Could you check a few things on this model? Use its own coordinates, in mm. A direction names the side the tool comes from. Round coordinates to 2 decimals unless told otherwise and drop trailing zeros. Loops run counter-clockwise (first coordinate to the right, second up) from the corner with the lowest first, then second, coordinate; pieces in that order, holes last. Notation, with made-up numbers: (1, -11) - (58, -11) arc R22 cw to (58, -1) - close; hole circle Ø11 at (20.25, 1). An arc over 180 degrees is marked (long way). Use one line per item in the form item = value.
```python
from build123d import *

# Parameters (mm, degrees)
SKETCH1_W           = 1300
SKETCH1_H           = 300
BOSS_EXTRUDE1_DEPTH = 700
FILLET1_R           = 200
FILLET2_R           = 100
FILLET3_R           = 100
FILLET4_R           = 100
SKETCH3_R           = 3.4
CUT_EXTRUDE1_DEPTH  = 100
CUT_EXTRUDE2_START  = -100
SKETCH4_R           = 3.4
CUT_EXTRUDE2_DEPTH  = 100
SKETCH5_W           = 631.976111166
SKETCH5_H           = 319.581114146
CUT_EXTRUDE4_DEPTH  = 1410
SKETCH6_W           = 352.69600487
SKETCH6_H           = 35.021102412
BOSS_EXTRUDE2_DEPTH = 631.976111165


with BuildPart() as part:
    # Sketch1 → Boss-Extrude1 (new body)
    with BuildSketch(Plane(origin=(0, 0, 0), x_dir=(-1, 0, 0), z_dir=(0, 1, 0))):
        Rectangle(SKETCH1_W, SKETCH1_H)
    extrude(amount=BOSS_EXTRUDE1_DEPTH)

    # Fillet1
    fillet1_edges = [part.edges().sort_by_distance(p)[0] for p in [
        (650, 350, 150),
    ]]
    fillet(fillet1_edges, radius=FILLET1_R)

    # Fillet2
    fillet2_edges = [part.edges().sort_by_distance(p)[0] for p in [
        (650, 350, -150),
    ]]
    fillet(fillet2_edges, radius=FILLET2_R - 0.0001)  # a hair under: the kernel refuses the full size

    # Fillet3
    fillet3_edges = [part.edges().sort_by_distance(p)[0] for p in [
        (-650, 350, 150),
    ]]
    fillet(fillet3_edges, radius=FILLET3_R)

    # Fillet4
    fillet4_edges = [part.edges().sort_by_distance(p)[0] for p in [
        (-650, 350, -150),
    ]]
    fillet(fillet4_edges, radius=FILLET4_R)

    # Sketch3 → Cut-Extrude1 (cut)
    with BuildSketch(Plane.XZ):
        with Locations(Location((475, 0, 0), (0, 0, 270))):
            Circle(SKETCH3_R)
        with Locations(Location((492.320508076, 10, 0), (0, 0, 270))):
            Circle(SKETCH3_R)
        with Locations(Location((457.679491924, 10, 0), (0, 0, 270))):
            Circle(SKETCH3_R)
        with Locations(Location((475, -20, 0), (0, 0, 270))):
            Circle(SKETCH3_R)
        with Locations(Location((-475, 0, 0), (0, 0, 270))):
            Circle(SKETCH3_R)
        with Locations(Location((-457.679491924, 10, 0), (0, 0, 270))):
            Circle(SKETCH3_R)
        with Locations(Location((-492.320508076, 10, 0), (0, 0, 270))):
            Circle(SKETCH3_R)
        with Locations(Location((-475, -20, 0), (0, 0, 270))):
            Circle(SKETCH3_R)
    extrude(amount=-CUT_EXTRUDE1_DEPTH, mode=Mode.SUBTRACT)

    # Sketch4 → Cut-Extrude2 (cut)
    with BuildSketch(Plane(origin=(0, 700, 0), x_dir=(-1, 0, 0), z_dir=(0, 1, 0)).offset(CUT_EXTRUDE2_START)):
        with Locations(Location((-475, 0, 0), (0, 0, 270))):
            Circle(SKETCH4_R)
        with Locations(Location((-475, 20, 0), (0, 0, 90))):
            Circle(SKETCH4_R)
        with Locations(Location((-492.320508076, -10, 0), (0, 0, 90))):
            Circle(SKETCH4_R)
        with Locations(Location((-457.679491924, -10, 0), (0, 0, 90))):
            Circle(SKETCH4_R)
        with Locations(Location((475, 0, 0), (0, 0, 270))):
            Circle(SKETCH4_R)
        with Locations(Location((475, 20, 0), (0, 0, 90))):
            Circle(SKETCH4_R)
        with Locations(Location((457.679491924, -10, 0), (0, 0, 90))):
            Circle(SKETCH4_R)
        with Locations(Location((492.320508076, -10, 0), (0, 0, 90))):
            Circle(SKETCH4_R)
    extrude(amount=CUT_EXTRUDE2_DEPTH, mode=Mode.SUBTRACT)

    # Sketch5 → Cut-Extrude4 (cut)
    with BuildSketch(Plane(origin=(-650, 0, 0), x_dir=(0, -1, 0), z_dir=(-1, 0, 0))):
        with Locations((-350, -43.959211894)):
            Rectangle(SKETCH5_W, SKETCH5_H)
    extrude(amount=-CUT_EXTRUDE4_DEPTH, mode=Mode.SUBTRACT)

    # Sketch6 → Boss-Extrude2 (add)
    with BuildSketch(Plane(origin=(0, 34.011944417, 0), x_dir=(-1, 0, 0), z_dir=(0, 1, 0))):
        with Locations((26.80489637, -132.489448794)):
            Rectangle(SKETCH6_W, SKETCH6_H)
    extrude(amount=BOSS_EXTRUDE2_DEPTH)


solid = part.part
```
1. We'd pull the mould along Y, two halves only. Please class faces 1 (the face through (8, 267, -150)), 2 (the face through (9, 0, 2)), 3 (the face through (-9, 665.988, -19)), 4 (the face through (9, 700, 2)): +Y half, -Y half, draft (parallel to the pull), parting line (faces both ways), or undercut.
Solution:
face_1 = draft
face_2 = -Y half
face_3 = undercut
face_4 = +Y half
2. For P1, Ø6, axis at x = -457.68, z = 10, coming from the -Y side; P2, Ø4, axis at x = 475, z = 0, coming from the -Y side; P3, Ø10.5, axis at y = 341.5, z = -125, coming from the -X side, each with a flat end and sliding along its axis, tell me the tip position at first contact or that it passes through.
Solution:
P1 = 665.99
P2 = through
P3 = -203.15
3. If we section it at D-D, the plane x = -168: Write out the boundary of the cut face in (y, z).
Solution:
outline = (0, -150) - (700, -150) - (700, 150) - (0, 150) - close; hole (34.01, -114.98) - (665.99, -114.98) - (665.99, 115.83) - (34.01, 115.83) - close
4. If we section it at C-C, the plane x = 301.5: Write out the boundary of the cut face in (y, z).
Solution:
outline = (0, -150) - (34.01, -150) - (34.01, 115.83) - (665.99, 115.83) - (665.99, -150) - (700, -150) - (700, 150) - (0, 150) - close
5. Please list where these lines run through material, in increasing order: line 1 along Z through (x, y) = (-475, 677.5); line 2 along Y through (x, z) = (341.5, 109); line 3 along X through (y, z) = (678.5, -10).
Solution:
line_1 = -150 to -3.4, 3.4 to 16.6, 23.4 to 150
line_2 = 0 to 34.01, 665.99 to 700
line_3 = -650 to -495.72, -488.92 to -461.08, -454.28 to 454.28, 461.08 to 488.92, 495.72 to 645.96
6. If we section it at B-B, the plane z = -97: Write out the boundary of the cut face in (x, y).
Solution:
outline = (-638.27, 0) - (638.27, 0) - (638.27, 34.01) - (-638.27, 34.01) - close; (-638.27, 665.99) - (638.27, 665.99) - (638.27, 700) - (-638.27, 700) - close
7. On a 3-axis mill with a long thin cutter (end or side, diameter ignored), from which of +Z, -Z, +X, -X, +Y, -Y can I reach the whole of each face in a straight line? I mean faces 5 (the face through (149.543, 346, -133)), 6 (the face through (-621.484, 17.244, -119.929)), 7 (the face through (-203.153, 346, -133)), 8 (the face through (-40, 354, 115.831)). Say none if no direction works.
Solution:
face_5 = -Z, +X
face_6 = -Z, -X, +Y, -Y
face_7 = -Z, -X
face_8 = +X, -X
8. If we section it at A-A, the plane y = 645: Write out the boundary of the cut face in (x, z), plus the area to 3 significant figures.
Solution:
outline = (-625.27, 115.83) - (561.8, 115.83) arc R200 ccw to (450, 150) - (-550, 150) arc R100 ccw to start; (-203.15, -150) - (149.54, -150) - (149.54, -114.98) - (-203.15, -114.98) - close
area = 50,900 mm^2
